Part print with two shaded views. Sizes in mm from the minimum x, y, z corner. Round coordinates to 2 decimals unless told otherwise and drop trailing zeros. Loops run counter-clockwise (first coordinate to the right, second up) from the corner with the lowest first, then second, coordinate; pieces in that order, holes last. Notation, with made-up numbers: (48.25, 69) -> (66.25, 69) arc R14 ccw to (66.25, 83) -> close; hole circle Ø9 at (22, 9.25). An arc over 180 degrees is marked (long way). Answer as a JSON object with one key per item and string values. Group by question number.
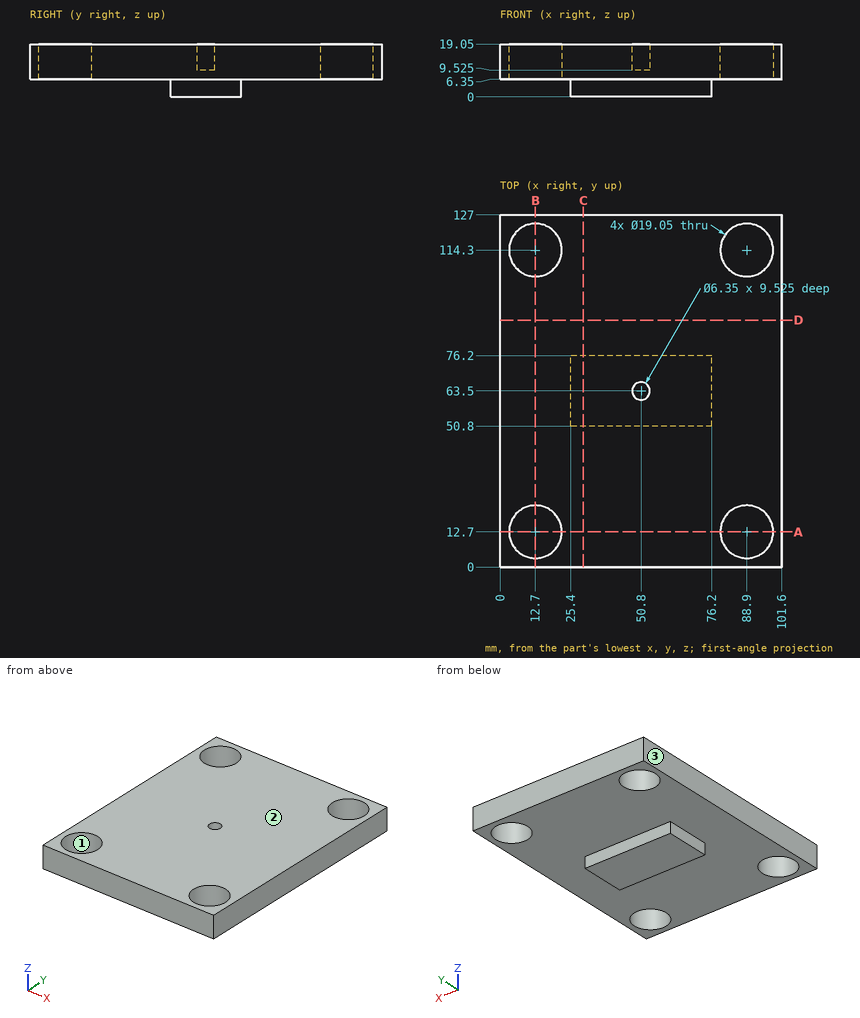
Item 1: Two-plate mould, pull along X, no slides. Class the marked faces 1, 2 and 3: pulls with the +X half, pulls with the -X half, needs draft (parallel to the pull), parting line crosses it, or undercut.
Item 2: Band-saw the part on C-C, the plane x = 30. List the corners of the cut face in (y, z), plus the area to 3 significant figures.
Item 3: Band-saw the part on B-B, the plane x = 12.7. List the corners of the cut face in (y, z) (3 decimals).
Item 4: Band-saw the part on D-D, the plane y = 89. List the corners of the cut face in (x, z).
Item 5: Band-saw the part on A-A, the plane y = 12.7. List the corners of the cut face in (x, z) (3 decimals).
Item 6: Drop flat-ended pins along their axis: pin 1 Ø3 at (y, z) = (61.5, 4) entering from +X; pin 2 Ø3 at (x, z) = (50.5, 3) entering from -Y; pin 3 Ø5 at (x, z) = (61, 15) entering from -Y; pin 4 Ø1 at (x, y) = (43.5, 27.5) entering from -Z. Give the stop position or say it passes through.
Item 7: Drill centre lines: line 1 (Y direction, x = 88.9, z = 16.25) (3 decimals); line 2 (Y direction, x = 50.8, z = 15) (3 decimals); line 3 (X direction, y = 121, z = 8.75). Where is each one in solid material? Low to high.
Entries:
{
 "1": {"face 1": "undercut", "face 2": "needs draft", "face 3": "pulls with the -X half"},
 "2": {"outline": "(0, 6.35) -> (50.8, 6.35) -> (50.8, 0) -> (76.2, 0) -> (76.2, 6.35) -> (127, 6.35) -> (127, 19.05) -> (0, 19.05) -> close", "area": "1,770 mm²"},
 "3": {"outline": "(0, 6.35) -> (3.175, 6.35) -> (3.175, 19.05) -> (0, 19.05) -> close; (22.225, 6.35) -> (104.775, 6.35) -> (104.775, 19.05) -> (22.225, 19.05) -> close; (123.825, 6.35) -> (127, 6.35) -> (127, 19.05) -> (123.825, 19.05) -> close"},
 "4": {"outline": "(0, 6.35) -> (101.6, 6.35) -> (101.6, 19.05) -> (0, 19.05) -> close"},
 "5": {"outline": "(0, 6.35) -> (3.175, 6.35) -> (3.175, 19.05) -> (0, 19.05) -> close; (22.225, 6.35) -> (79.375, 6.35) -> (79.375, 19.05) -> (22.225, 19.05) -> close; (98.425, 6.35) -> (101.6, 6.35) -> (101.6, 19.05) -> (98.425, 19.05) -> close"},
 "6": {"pin 1": "x = 76.2", "pin 2": "y = 50.8", "pin 3": "y = 0", "pin 4": "z = 6.35"},
 "7": {"line 1": "0 to 3.175, 22.225 to 104.775, 123.825 to 127", "line 2": "0 to 60.325, 66.675 to 127", "line 3": "0 to 5.93, 19.47 to 82.13, 95.67 to 101.6"}
}
